For this review, take the finished solid that the model builds, in its own axes (mm). A direction names the side the tool comes from. Coordinates: 2 decimals unless noted, no trailing zeros. Loops run counter-clockwise (first coordinate to the right, second up) from the corner with the lowest first, then second, coordinate; pieces in that order, holes last. Notation, with made-up numbers: (2.5, 73) - (41.5, 73) arc R27 ccw to (41.5, 96) - close; hole circle Ø2 at (30.5, 59.25). An arc over 180 degrees is marked (long way). Use one line per item in the form item = value. Start each with the question number.
1. Add section D-D on x = 27. Give the boundary of the cut face in (y, z), and give its area (3 significant figures).
2. Add section B-B on y = 57.15. Give the boundary of the cut face in (x, z).
3. Add section C-C on x = 4. Give the boundary of the cut face in (y, z), and give its area (3 significant figures).
4. Draft analysis for pull direction Z (two halves, no side actions). For faces 4 (the face through (-23, 65.088, -24)), 5 (the face through (-35, 15.875, 5)), 6 (the face through (-15, 32, -31.081)), state which applies: +Z half, -Z half, draft (parallel to the pull), parting line (faces both ways), or undercut.
5. Add section A-A on z = -2. Give the boundary of the cut face in (x, y) (1 decimal).
6. For pin 1 Ø4.5 at (x, y) = (27.53, 57.15) entering from -Z; pin 2 Ø12 at (y, z) = (25, 23) entering from +X; pin 3 Ø10 at (x, y) = (23.5, 57) entering from +Z, all flat-tipped, find the tip position at first contact; note any pin that passes through.
7. Machinability: for faces 1 (the face through (-35, 49.212, 5)), 2 (the face through (-25, 63.5, -26)), 3 (the face through (-22.608, 55.376, -32.691)), which of the approach directions +Z, -Z, +X, -X, +Y, -Y give a long, thin tool a straight path to every point of the face, cutting with its end or side? Answer none if there is none.
8. To check wall thickness, follow probe 1 along Z at (x, y) = (10, 48); probe 2 along X at (y, z) = (27.5, 22.5). State the ranges of each line that lie inside material, in increasing order.
```python
from build123d import *

# Parameters (mm, degrees)
BOSS_EXTRUDE1_DEPTH = 65.0875
SKETCH2_R           = 2
SKETCH2_R_2         = 12.7
CUT_EXTRUDE1_DEPTH  = 3.175
CUT_EXTRUDE2_DEPTH  = 3.175
BOSS_EXTRUDE2_START = -1.5875
BOSS_EXTRUDE2_DEPTH = 1.5875
CUT_EXTRUDE3_DEPTH  = 3.175


with BuildPart() as part:
    # Sketch1 → Boss-Extrude1 (new body)
    with BuildSketch(Plane(origin=(0, 0, 0), x_dir=(1, 0, 0), z_dir=(0, 1, 0))):
        with BuildLine():
            Line((32.013617701, 34.255816606), (32.013617701, 31.080816606))
            Line((32.013617701, 31.080816606), (-33.073882299, 31.080816606))
            Line((-33.073882299, 31.080816606), (-33.073882299, -34.006683394))
            Line((-33.073882299, -34.006683394), (-36.248882299, -34.006683394))
            Line((-36.248882299, -34.006683394), (-36.248882299, 31.715816606))
            ThreePointArc((-36.248882299, 31.715816606), (-35.504933523, 33.51186783), (-33.708882299, 34.255816606))
            Line((-33.708882299, 34.255816606), (32.013617701, 34.255816606))
        make_face()
    extrude(amount=BOSS_EXTRUDE1_DEPTH)

    # Sketch2 → Cut-Extrude1 (cut)
    with BuildSketch(Plane(origin=(0, 0, -34.255816606), x_dir=(-1, 0, 0), z_dir=(0, 0, -1))):
        with Locations((-27.52729049, 57.15)):
            Circle(SKETCH2_R)
        with Locations((21.68520951, 57.15)):
            Circle(SKETCH2_R)
        with Locations((21.68520951, 7.9375)):
            Circle(SKETCH2_R)
        with Locations((-27.52729049, 7.9375)):
            Circle(SKETCH2_R)
        with Locations((-2.92104049, 32.54375)):
            Circle(SKETCH2_R_2)
        Polygon((-29.473617701, 65.0875), (-32.013617701, 62.5475), (-32.013617701, 65.0875), align=None)
        Polygon((-29.473617701, 0), (-32.013617701, 2.54), (-32.013617701, 0), align=None)
    extrude(amount=-CUT_EXTRUDE1_DEPTH, mode=Mode.SUBTRACT)

    # Sketch3 → Cut-Extrude2 (cut)
    with BuildSketch(Plane.ZY.offset(36.248882299)):
        with BuildLine():
            Line((27.656683394, 65.0875), (34.006683394, 65.0875))
            Line((34.006683394, 65.0875), (34.006683394, 58.7375))
            ThreePointArc((34.006683394, 58.7375), (32.146811455, 63.227628061), (27.656683394, 65.0875))
        make_face()
        with BuildLine():
            Line((34.006683394, 6.35), (34.006683394, 0))
            Line((34.006683394, 0), (27.656683394, 0))
            ThreePointArc((27.656683394, 0), (32.146811455, 1.859871939), (34.006683394, 6.35))
        make_face()
    extrude(amount=-CUT_EXTRUDE2_DEPTH, mode=Mode.SUBTRACT)

    # Sketch4 → Boss-Extrude2 (add)
    with BuildSketch(Plane(origin=(0, 65.0875, 0), x_dir=(1, 0, 0), z_dir=(0, 1, 0)).offset(BOSS_EXTRUDE2_START)):
        with BuildLine():
            Line((-36.248882299, 31.715816606), (-36.248882299, 15.205816606))
            Line((-36.248882299, 15.205816606), (-6.086382299, 34.255816606))
            Line((-6.086382299, 34.255816606), (-33.708882299, 34.255816606))
            ThreePointArc((-33.708882299, 34.255816606), (-35.504933523, 33.51186783), (-36.248882299, 31.715816606))
        make_face()
    boss_extrude2 = extrude(amount=BOSS_EXTRUDE2_DEPTH)

    # Mirror1: Boss-Extrude2 across plane
    add(boss_extrude2.mirror(Plane(origin=(0, 32.54375, 0), x_dir=(0, 0, 1), z_dir=(0, -1, 0))))

    # Sketch5 → Cut-Extrude3 (cut)
    with BuildSketch(Plane.ZY.offset(36.248882299)):
        with BuildLine():
            Line((-17.250449478, 53.975), (27.199550522, 53.975))
            ThreePointArc((27.199550522, 53.975), (29.580800522, 51.59375), (27.199550522, 49.2125))
            Line((27.199550522, 49.2125), (-17.250449478, 49.2125))
            ThreePointArc((-17.250449478, 49.2125), (-19.631699478, 51.59375), (-17.250449478, 53.975))
        make_face()
        with BuildLine():
            Line((-17.250449478, 11.1125), (27.199550522, 11.1125))
            ThreePointArc((27.199550522, 11.1125), (29.580800522, 13.49375), (27.199550522, 15.875))
            Line((27.199550522, 15.875), (-17.250449478, 15.875))
            ThreePointArc((-17.250449478, 15.875), (-19.631699478, 13.49375), (-17.250449478, 11.1125))
        make_face()
    extrude(amount=-CUT_EXTRUDE3_DEPTH, mode=Mode.SUBTRACT)


solid = part.part
```
Conclusion:
q1.outline = (0, -34.26) - (6.01, -34.26) - (6.01, -31.08) - (0, -31.08) - close; (9.87, -34.26) - (55.22, -34.26) - (55.22, -31.08) - (9.87, -31.08) - close; (59.08, -34.26) - (65.09, -34.26) - (65.09, -31.08) - (59.08, -31.08) - close
q1.area = 182 mm^2
q2.outline = (-36.25, -31.72) arc R2.54 ccw to (-33.71, -34.26) - (-23.69, -34.26) - (-23.69, -31.08) - (-33.07, -31.08) - (-33.07, 34.01) - (-36.25, 34.01) - close; (-19.69, -34.26) - (25.53, -34.26) - (25.53, -31.08) - (-19.69, -31.08) - close; (29.53, -34.26) - (32.01, -34.26) - (32.01, -31.08) - (29.53, -31.08) - close
q3.outline = (0, -34.26) - (19.89, -34.26) - (19.89, -31.08) - (0, -31.08) - close; (45.2, -34.26) - (65.09, -34.26) - (65.09, -31.08) - (45.2, -31.08) - close
q3.area = 126 mm^2
q4.face_4 = draft
q4.face_5 = undercut
q4.face_6 = +Z half
q5.outline = (-36.2, 0) - (-33.1, 0) - (-33.1, 11.1) - (-36.2, 11.1) - close; (-36.2, 15.9) - (-33.1, 15.9) - (-33.1, 49.2) - (-36.2, 49.2) - close; (-36.2, 54) - (-33.1, 54) - (-33.1, 65.1) - (-36.2, 65.1) - close
q6.pin_1 = -34.26
q6.pin_2 = -33.07
q6.pin_3 = -31.08
q7.face_1 = +X, -X
q7.face_2 = +Z, +X
q7.face_3 = +Z, -Z
q8.probe_1 = -34.26 to -31.08
q8.probe_2 = -36.25 to -33.07
